from build123d import *

# Parameters (mm, degrees)
CROQUIS1_W              = 140
CROQUIS1_H              = 140
CROQUIS1_R              = 1.5
CROQUIS1_W_2            = 110
CROQUIS1_H_2            = 110
SALIENTE_EXTRUIR1_DEPTH = 5
CROQUIS2_W              = 5
CROQUIS2_H              = 10
CORTAR_EXTRUIR1_DEPTH   = 5


with BuildPart() as part:
    # Croquis1 → Saliente-Extruir1 (new body)
    with BuildSketch(Plane(origin=(0, 0, 0), x_dir=(1, 0, 0), z_dir=(0, 1, 0))):
        Rectangle(CROQUIS1_W, CROQUIS1_H)
        with Locations(Location((-61, 61, 0), (0, 0, 270))):
            Circle(CROQUIS1_R, mode=Mode.SUBTRACT)
        with Locations(Location((66, 61, 0), (0, 0, 270))):
            Circle(CROQUIS1_R, mode=Mode.SUBTRACT)
        with Locations(Location((66, -61, 0), (0, 0, 270))):
            Circle(CROQUIS1_R, mode=Mode.SUBTRACT)
        with Locations(Location((-61, -61, 0), (0, 0, 270))):
            Circle(CROQUIS1_R, mode=Mode.SUBTRACT)
        with Locations(Location((66, 30.5, 0), (0, 0, 270))):
            Circle(CROQUIS1_R, mode=Mode.SUBTRACT)
        with Locations(Location((66, -30.5, 0), (0, 0, 270))):
            Circle(CROQUIS1_R, mode=Mode.SUBTRACT)
        with Locations(Location((-30.5, -66, 0), (0, 0, 270))):
            Circle(CROQUIS1_R, mode=Mode.SUBTRACT)
        with Locations(Location((30.5, -66, 0), (0, 0, 270))):
            Circle(CROQUIS1_R, mode=Mode.SUBTRACT)
        with Locations(Location((-30.5, 66, 0), (0, 0, 90))):
            Circle(CROQUIS1_R, mode=Mode.SUBTRACT)
        with Locations(Location((30.5, 66, 0), (0, 0, 90))):
            Circle(CROQUIS1_R, mode=Mode.SUBTRACT)
        with Locations(Location((-66, 30.5, 0), (0, 0, 90))):
            Circle(CROQUIS1_R, mode=Mode.SUBTRACT)
        with Locations(Location((-66, -30.5, 0), (0, 0, 90))):
            Circle(CROQUIS1_R, mode=Mode.SUBTRACT)
        Rectangle(CROQUIS1_W_2, CROQUIS1_H_2, mode=Mode.SUBTRACT)
    extrude(amount=SALIENTE_EXTRUIR1_DEPTH)

    # Croquis2 → Cortar-Extruir1 (cut)
    with BuildSketch(Plane(origin=(0, 5, 0), x_dir=(1, 0, 0), z_dir=(0, 1, 0))):
        with Locations((60, -50)):
            Rectangle(CROQUIS2_W, CROQUIS2_H)
        with Locations((-60, -50)):
            Rectangle(CROQUIS2_W, CROQUIS2_H)
    extrude(amount=-CORTAR_EXTRUIR1_DEPTH, mode=Mode.SUBTRACT)


solid = part.part
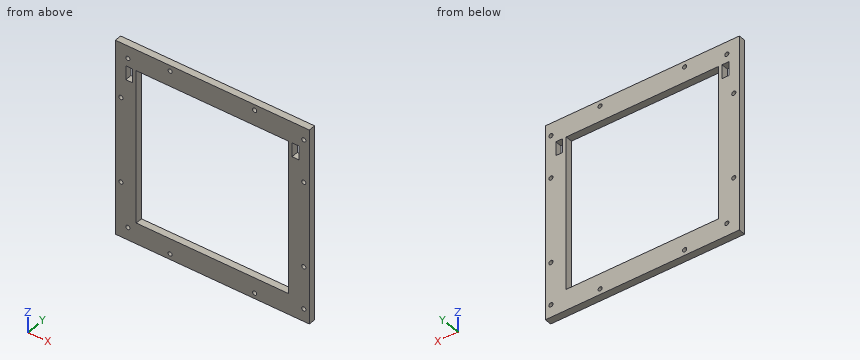
CAD build for the part. Positions are in the model's coordinates, mm. Round coordinates to 2 decimals unless told otherwise and drop trailing zeros. Loops run counter-clockwise (first coordinate to the right, second up) from the corner with the lowest first, then second, coordinate; pieces in that order, holes last. Notation, with made-up numbers: (61, 60.25) - (90, 60.25) arc R14 cw to (90, 72.25) - close; hole circle Ø6 at (29.25, -7). An arc over 180 degrees is marked (long way). Put each result on its own line as item: value.
1. Slice it at B-B on x = 2.5. List the corners of the cut face in (y, z).
Geometry check:
outline: (0, -70) - (5, -70) - (5, -55) - (0, -55) - close; (0, 55) - (5, 55) - (5, 70) - (0, 70) - close
2. Slice it at C-C on y = 4. Give the number of separate pieces and of enclosed holes in the cut face, and give its area (3 significant figures).
Geometry check:
separate pieces: 1
enclosed holes: 15
area: 7,320 mm²
3. Slice it at A-A on z = 39. List the corners of the cut face in (x, y), and give its area (3 significant figures).
Geometry check:
outline: (-70, 0) - (-55, 0) - (-55, 5) - (-70, 5) - close; (55, 0) - (70, 0) - (70, 5) - (55, 5) - close
area: 150 mm²
4. Wall check: line 1 (Z direction, x = -66, y = 2.85); line 2 (X direction, y = 2.9, z = 52); line 3 (Z direction, x = -25.5, y = 4.6). Give the ranges that are in metal, low to high.
Geometry check:
line 1: -70 to -32, -29 to 29, 32 to 70
line 2: -70 to -62.5, -57.5 to -55, 55 to 57.5, 62.5 to 70
line 3: -70 to -55, 55 to 70
